Design review of the part shown in the three views and the two pictorial views. Dimensions are in mm from the part's minimum x, y and z. A direction names the side the tool comes from. Round coordinates to 2 decimals unless told otherwise and drop trailing zeros. Order: outer loops, then holes, each group sorted by start corner. A loop starts at its lowest first (then second) coordinate and runs counter-clockwise, first axis right, second up. Notation, with made-up numbers: (-4, 79) - (48, 79) arc R28 ccw to (48, 103) - close; hole circle Ø3 at (29.5, 39.5). An arc over 180 degrees is marked (long way). One line per item, written item: value.
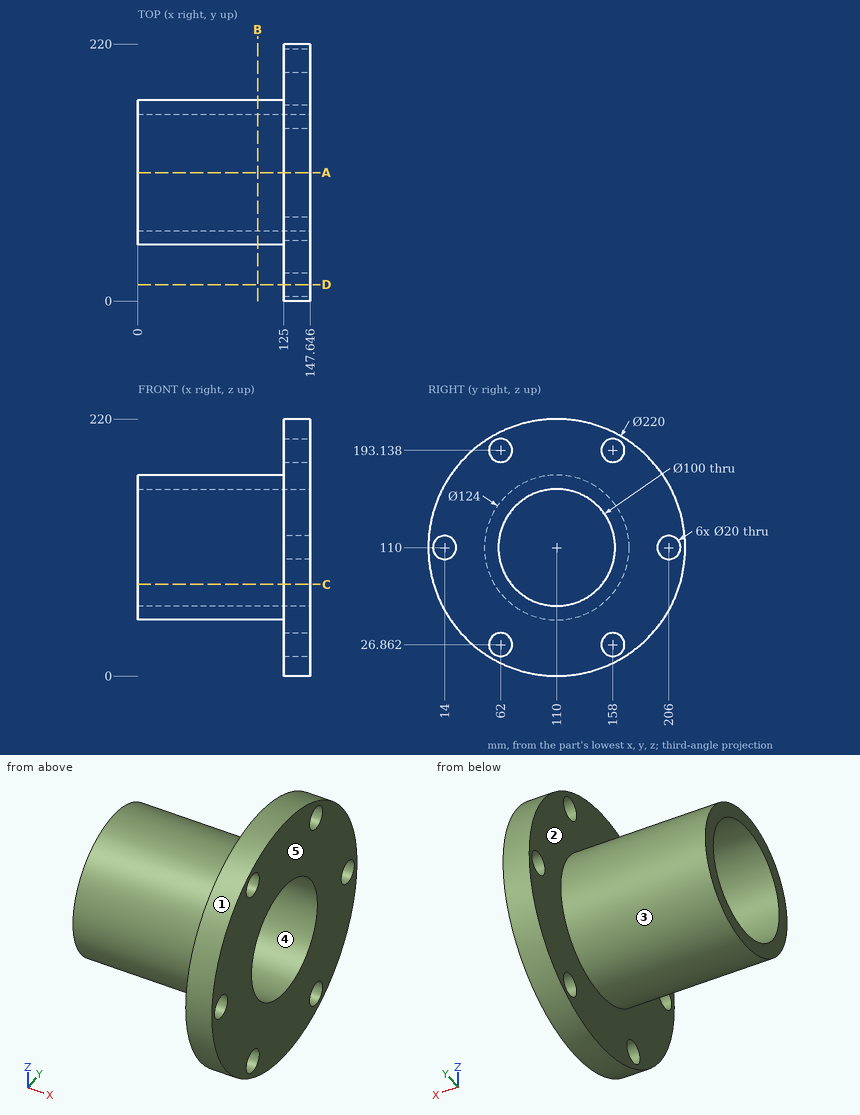
Item 1: The part is to be moulded in two halves that separate along Y. For the marked faces 3, 4 and 5, say which applies: +Y half, -Y half, draft (parallel to the pull), parting line (faces both ways), or undercut.
Returned:
face 3: parting line
face 4: undercut
face 5: draft
Item 2: For P1, Ø1, axis at y = 63.5, z = 64.5, coming from the -X side; P2, Ø10, axis at y = 66, z = 155, coming from the -X side; P3, Ø8, axis at x = 91.5, z = 55.5, coming from the +Y side; P4, Ø8, axis at x = 19.5, y = 99, coming from the +Z side, all flat-tipped, find the tip position at first contact; note any pin that passes through.
Returned:
P1: x = 125
P2: x = 0
P3: y = 145.97
P4: z = 171.6
Item 3: Take a section at C-C (z = 78.5). Write out the cut boundary in (x, y) (1 decimal), plus the area to 3 significant figures.
Returned:
outline: (0, 56.6) - (125, 56.6) - (125, 4.6) - (147.6, 4.6) - (147.6, 71.2) - (0, 71.2) - close; (0, 148.8) - (147.6, 148.8) - (147.6, 215.4) - (125, 215.4) - (125, 163.4) - (0, 163.4) - close
area: 6,660 mm^2
Item 4: Wall thickness on line 1 (Z direction, x = 51, y = 110); line 2 (X direction, y = 197.5, z = 86) (1 decimal); line 3 (Z direction, x = 130.5, y = 58.5) (1 decimal): over which ranges is each line inside the solid? List them lowest first.
Returned:
line 1: 48 to 60, 160 to 172
line 2: 125 to 147.6
line 3: 12.8 to 17.5, 36.2 to 183.8, 202.5 to 207.2
Item 5: Take a section at B-B (x = 102.5). Write out the cut boundary in (y, z), plus the area to 3 significant figures.
Returned:
outline: circle Ø124 at (110, 110); hole circle Ø100 at (110, 110)
area: 4,220 mm^2
Item 6: Machinability: for the marked faces 1 and 2, which of the approach directions +Z, -Z, +X, -X, +Y, -Y give a long, thin tool a straight path to every point of the face, cutting with its end or side? Answer none if there is none.
Returned:
face 1: +X, -X
face 2: -X
Item 7: Take a section at A-A (y = 110). Write out the cut boundary in (x, z) (1 decimal).
Returned:
outline: (0, 48) - (125, 48) - (125, 0) - (147.6, 0) - (147.6, 60) - (0, 60) - close; (0, 160) - (147.6, 160) - (147.6, 220) - (125, 220) - (125, 172) - (0, 172) - close
Item 8: Take a section at D-D (y = 14). Write out the cut boundary in (x, z) (1 decimal).
Returned:
outline: (125, 56.3) - (147.6, 56.3) - (147.6, 100) - (125, 100) - close; (125, 120) - (147.6, 120) - (147.6, 163.7) - (125, 163.7) - close
